The listing builds one solid part. Answer for the finished solid, in the listing's coordinates (mm). Give positions to 0.01 mm unless a question says otherwise; leave off trailing zeros.
Item 1: Each of these flat-tipped pins is pushed along its axis until it touches: pin 1 Ø9 at (x, y) = (-12.7, 0) entering from -Z; pin 2 Ø16.5 at (x, y) = (-27.5, -15.87) entering from -Z. Where does it stop, or does it pass through?
Item 2: Consider line 1 along Y through (x, z) = (-67, 0.4); line 2 along X through (y, z) = (-46.5, 1.8); line 3 along Y through (x, z) = (-13.5, 1.9). Determine where each line is inside the solid, lowest interval first.
Item 3: Section A-A, the plane x = 0 is taken. Give the number of separate pieces and of enclosed holes in the cut face, and give its area (3 significant figures).
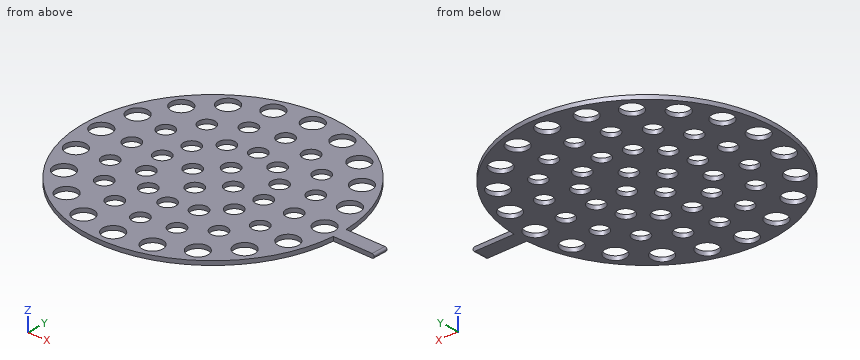
from build123d import *

# Parameters (mm, degrees)
F1_DEPTH         = 2.54
F4_R             = 5.08
F5_DEPTH         = 25.4
F5_COPIES_COUNT  = 16
F6_R             = 6.35
F8_DEPTH         = 25.4
F8_COPIES_COUNT  = 20
F3_R             = 5.08
F9_DEPTH         = 25.4
F9_COPIES_COUNT  = 12
F2_R             = 5.08
F10_DEPTH        = 25.4
F10_COPIES_COUNT = 4
F11_R            = 1.26999


# Not quite as in the source:
# - a fillet or chamfer is up to 0.001 mm smaller than in the source, because OpenCascade refuses the exact size
# - a pattern or mirror of a feature is missing from the dataset's text; its kind, count and spacing are read off the source's solid


with BuildPart() as f1:
    # F0 (on Top) → F1 (new body)
    with BuildSketch(Plane.XY):
        with BuildLine():
            ThreePointArc((79.2488887438, -4.4726119748), (79.343465922, -2.2371947795), (79.375, 0))
            ThreePointArc((79.375, 0), (79.343465922, 2.2371947795), (79.2488887438, 4.4726119748))
            Line((79.2488887438, 4.4726119748), (79.2488887438, -4.4726119748))
        make_face()
        with BuildLine():
            ThreePointArc((79.2488887438, 4.4726119748), (79.343465922, 2.2371947795), (79.375, 0))
            ThreePointArc((79.375, 0), (79.343465922, -2.2371947795), (79.2488887438, -4.4726119748))
            Line((79.2488887438, -4.4726119748), (104.8729870915, -4.4726119748))
            Line((104.8729870915, -4.4726119748), (104.8729870915, 4.4726119748))
            Line((104.8729870915, 4.4726119748), (79.2488887438, 4.4726119748))
        make_face()
        with BuildLine():
            Line((79.2488887438, -4.4726119748), (79.2488887438, 4.4726119748))
            ThreePointArc((79.2488887438, 4.4726119748), (-79.375, 0), (79.2488887438, -4.4726119748))
        make_face()
    extrude(amount=F1_DEPTH)

    # F4 (on Top) → F5 (cut)
    with BuildSketch(Plane.XY):
        with Locations((0, 50.8)):
            Circle(F4_R)
    f5 = extrude(amount=F5_DEPTH, mode=Mode.SUBTRACT)

    # F5_copies: F5 ×16 about axis
    f5_copies_axis = Axis((0, 0, 0), (0, 0, 1))
    for i in range(1, F5_COPIES_COUNT):
        add(f5.rotate(f5_copies_axis, i * 360 / F5_COPIES_COUNT), mode=Mode.SUBTRACT)

    # F6 (on Top) → F8 (cut)
    with BuildSketch(Plane.XY):
        with Locations((0, 69.85)):
            Circle(F6_R)
    f8 = extrude(amount=F8_DEPTH, mode=Mode.SUBTRACT)

    # F8_copies: F8 ×20 about axis
    f8_copies_axis = Axis((0, 0, 0), (0, 0, 1))
    for i in range(1, F8_COPIES_COUNT):
        add(f8.rotate(f8_copies_axis, i * 360 / F8_COPIES_COUNT), mode=Mode.SUBTRACT)

    # F3 (on Top) → F9 (cut)
    with BuildSketch(Plane.XY):
        with Locations((0, 31.75)):
            Circle(F3_R)
    f9 = extrude(amount=F9_DEPTH, mode=Mode.SUBTRACT)

    # F9_copies: F9 ×12 about axis
    f9_copies_axis = Axis((0, 0, 0), (0, 0, 1))
    for i in range(1, F9_COPIES_COUNT):
        add(f9.rotate(f9_copies_axis, i * 360 / F9_COPIES_COUNT), mode=Mode.SUBTRACT)

    # F2 (on Top) → F10 (cut)
    with BuildSketch(Plane.XY):
        with Locations((0, 12.7)):
            Circle(F2_R)
    f10 = extrude(amount=F10_DEPTH, mode=Mode.SUBTRACT)

    # F10_copies: F10 ×4 about axis
    f10_copies_axis = Axis((0, 0, 0), (0, 0, 1))
    for i in range(1, F10_COPIES_COUNT):
        add(f10.rotate(f10_copies_axis, i * 360 / F10_COPIES_COUNT), mode=Mode.SUBTRACT)

    # F11 (radius 1.27 in the source; OpenCascade refuses exactly that, so slightly less here)
    f11_edges = [f1.edges().sort_by_distance(p)[0] for p in [
        (104.872987, 0, 0),
        (104.872987, 0, 2.54),
    ]]
    fillet(f11_edges, radius=F11_R)


solid = f1.part
Worked answers:
1. pin 1: passes through
1. pin 2: stops at z = 0
2. line 1: y = -42.56 to -27.91, -15.26 to -5.67, 5.67 to 15.26, 27.91 to 42.56
2. line 2: x = -64.33 to -59.78, -53.24 to -24.5, -14.38 to -2.7, 2.7 to 14.38, 24.5 to 53.24, 59.78 to 64.33
2. line 3: y = -78.22 to -31.99, -23.01 to -5.02, 5.02 to 23.01, 31.99 to 78.22
3. separate pieces: 9
3. enclosed holes: 0
3. area: 184 mm2
